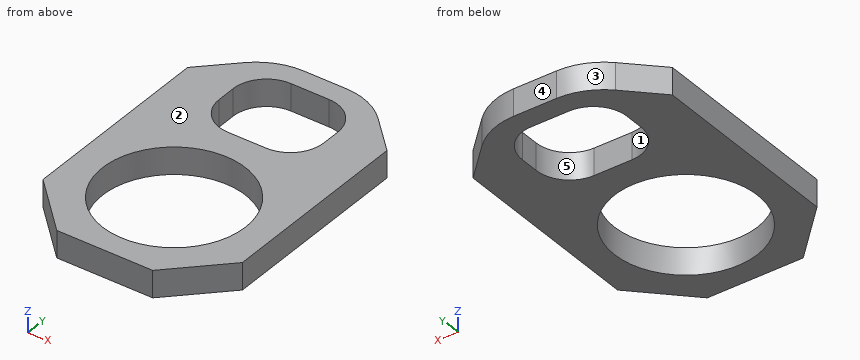
from build123d import *

# Parameters (mm, degrees)
F0_R     = 16.8529
F1_DEPTH = 6.35


with BuildPart() as f1:
    # F0 (on Top) → F1 (new body)
    with BuildSketch(Plane.XY):
        with BuildLine():
            Line((0, 12.192), (12.192, 0))
            Line((12.192, 0), (34.798, 0))
            Line((34.798, 0), (46.99, 12.192))
            Line((46.99, 12.192), (46.99, 58.674))
            Line((46.99, 58.674), (39.25383, 66.345702))
            ThreePointArc((39.25383, 66.345702), (34.325333, 69.616494), (28.522706, 70.7644))
            Line((28.522706, 70.7644), (18.467294, 70.7644))
            ThreePointArc((18.467294, 70.7644), (12.664667, 69.616494), (7.73617, 66.345702))
            Line((7.73617, 66.345702), (0, 58.674))
            Line((0, 58.674), (0, 12.192))
        make_face()
        with Locations((23.622, 22.098)):
            Circle(F0_R, mode=Mode.SUBTRACT)
        with BuildLine():
            ThreePointArc((11.176, 58.0644), (13.482241, 63.632159), (19.05, 65.9384))
            Line((19.05, 65.9384), (27.94, 65.9384))
            ThreePointArc((27.94, 65.9384), (33.507759, 63.632159), (35.814, 58.0644))
            Line((35.814, 58.0644), (35.814, 53.594))
            ThreePointArc((35.814, 53.594), (33.507759, 48.026241), (27.94, 45.72))
            Line((27.94, 45.72), (19.05, 45.72))
            ThreePointArc((19.05, 45.72), (13.482241, 48.026241), (11.176, 53.594))
            Line((11.176, 53.594), (11.176, 58.0644))
        make_face(mode=Mode.SUBTRACT)
    extrude(amount=F1_DEPTH)


solid = f1.part
Source: CAD feature listing. Evaluate the final solid. Frame: model axes, mm. Face numbers are marked on the shaded views. A direction names the side the tool comes from. Give positions to 0.01 mm unless a question says otherwise; leave off trailing zeros. Write each loop counter-clockwise with the first axis right and the second up, starting at its lowest first coordinate (ties: lowest second). Pieces come first, ordered by that corner, then holes. Notation, with made-up numbers: (13.25, 73.25) -> (35.25, 73.25) arc R8 cw to (35.25, 81.25) -> close; hole circle Ø1 at (89, -4.5). An arc over 180 degrees is marked (long way). Write item = value, one per line.
Q1. Cut plane C-C on z = 1.25. Return loops of the section in (x, y).
Here are the results:
outline = (0, 12.19) -> (12.19, 0) -> (34.8, 0) -> (46.99, 12.19) -> (46.99, 58.67) -> (39.25, 66.35) arc R15.24 ccw to (28.52, 70.76) -> (18.47, 70.76) arc R15.24 ccw to (7.74, 66.35) -> (0, 58.67) -> close; hole circle Ø33.71 at (23.62, 22.1); hole (11.18, 53.59) arc R7.87 ccw to (19.05, 45.72) -> (27.94, 45.72) arc R7.87 ccw to (35.81, 53.59) -> (35.81, 58.06) arc R7.87 ccw to (27.94, 65.94) -> (19.05, 65.94) arc R7.87 ccw to (11.18, 58.06) -> close
Q2. Cut plane A-A on y = 16. Return loops of the section in (x, z).
Here are the results:
outline = (0, 0) -> (7.91, 0) -> (7.91, 6.35) -> (0, 6.35) -> close; (39.33, 0) -> (46.99, 0) -> (46.99, 6.35) -> (39.33, 6.35) -> close
Q3. Cut plane B-B on x = 30. Return loops of the section in (y, z).
Here are the results:
outline = (0, 0) -> (6.5, 0) -> (6.5, 6.35) -> (0, 6.35) -> close; (37.7, 0) -> (45.99, 0) -> (45.99, 6.35) -> (37.7, 6.35) -> close; (65.66, 0) -> (70.69, 0) -> (70.69, 6.35) -> (65.66, 6.35) -> close
Q4. Reachability of the marked faces 4 and 5 from +Z, -Z, +X, -X, +Y, -Y: full face, straight path, thin tool, end or side. Return the list, or none.
Here are the results:
face_4 = +Z, -Z, +X, -X, +Y
face_5 = +Z, -Z
Q5. Cut plane D-D on y = 25.5. Return loops of the section in (x, z).
Here are the results:
outline = (0, 0) -> (7.12, 0) -> (7.12, 6.35) -> (0, 6.35) -> close; (40.13, 0) -> (46.99, 0) -> (46.99, 6.35) -> (40.13, 6.35) -> close
Q6. First-contact query: pin 1 (3 mm diameter, centred on y = 40.5, z = 5.5, fed in from -X); pin 2 (1 mm diameter, centred on x = 27.5, y = 48, fed in from +Z). Flat tips, straight axial feed; report the tip coordinate or a pass-through.
Here are the results:
pin_1 = 0
pin_2 = through
Q7. Mould query, pull axis Y, two halves, no side actions, for the marked faces 1, 2 and 3. Classes: +Y half, -Y half, draft (parallel to the pull), parting line (faces both ways), or undercut.
Here are the results:
face_1 = undercut
face_2 = draft
face_3 = +Y half
Q8. Line query: line 1 (Y direction, x = 13, z = 3.75); line 2 (Y direction, x = 18, z = 1); line 3 (X direction, y = 25, z = 1.25). Output: solid intervals per line, ascending. Write a range as from..to.
Here are the results:
line_1 = 0..9.01, 35.18..48.55, 63.1..69.75
line_2 = 0..6.21, 37.99..45.79, 65.87..70.76
line_3 = 0..7.02, 40.22..46.99
